CAD build for the part. Positions are in the model's coordinates, mm. Face numbers are marked on the shaded views. Coordinates: 2 decimals unless noted, no trailing zeros. Loops run counter-clockwise (first coordinate to the right, second up) from the corner with the lowest first, then second, coordinate; pieces in that order, holes last. Notation, with made-up numbers: (-33, -11) - (-29, -11) arc R22 cw to (-29, 4) - close; hole circle Ø10 at (8, 27). An arc over 180 degrees is marked (long way). Put each result on its own line as item: value.
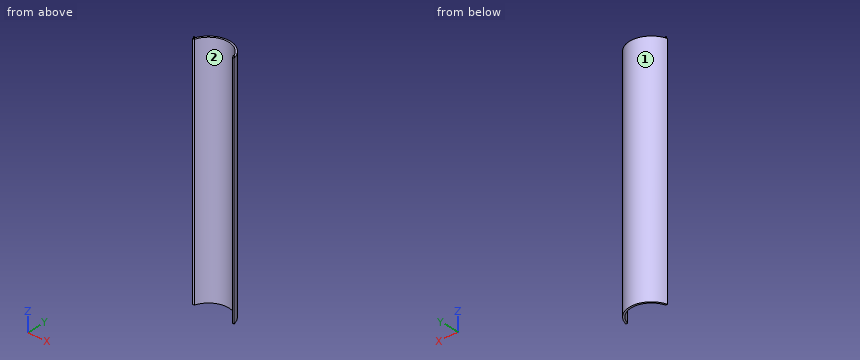
Autodesk Inventor part; units mm, degrees
ref_plane "YZ Plane" through (0, 0, 0) normal (1, 0, 0) x (0, 1, 0)
ref_plane "XZ Plane" through (0, 0, 0) normal (0, 1, 0) x (-1, 0, 0)
ref_plane "XY Plane" through (0, 0, 0) normal (0, 0, 1) x (1, 0, 0)
sketch "Sketch1" plane through (0, 0, 0) normal (0, 0, 1) x (1, 0, 0)
  circle A0 centre (0, 0) radius 25.4
  circle A1 centre (0, 0) radius 23.4
  dimension "d0" = 50.8
  dimension "d1" = 2
extrude "Extrusion1" add sketch "Sketch1" against normal blind 274
sketch "Sketch2" plane through (0, 0, 0) normal (0, 0, 1) x (1, 0, 0)
  line L0 (-25.4, 6.35) -> (25.4, 6.35)
  line L1 (25.4, 6.35) -> (25.4, -25.4)
  line L2 (25.4, -25.4) -> (-25.4, -25.4)
  line L3 (-25.4, -25.4) -> (-25.4, 6.35)
  circle A0 centre (0, 0) radius 25.4
  line L4 (0, 25.4) -> (0, -25.4)
  point P0 (-24.5934, 6.35)
  point P1 (24.5934, 6.35)
  dimension "d6" = 25.4
  dimension "d7" = 25.4
  dimension "d8" = 25.4
  dimension "d9" = 19.05
extrude "Extrusion2" cut sketch "Sketch2" against normal through all contours L0 L4 A0 | L0 A0 L4 picked at (-1.884, -14.6044) picked at (1.884, -14.6044)
sketch "Sketch3" plane through (0, 0, 0) normal (0, 0, 1) x (1, 0, 0)
  line L0 (22.5219, 6.35) -> (24.5934, 6.35)
  line L1 (23.5577, 6.35) -> (23.5577, 9.4971)
  arc A0 (24.5934, 6.35) -> (-24.5934, 6.35) centre (0, 0) ccw
  circle A1 centre (23.5577, 6.85) radius 0.5
  line L2 (0, 25.4) -> (0, 6.35) construction
  circle A2 centre (-23.5577, 6.85) radius 0.5
  dimension "d12" = 1
  dimension "d13" = 0.5
extrude "Extrusion3" add sketch "Sketch3" along normal blind 2 contours A1 L1 | L1 A1 | A2
properties part number "PCB Tray Top_3DPrint"
Q1. Slice it at A-A, the plane y = 20. Give the cut face in (x, z), then the cut area to 3 significant figures.
Determined:
outline: (-15.66, -274) - (-12.15, -274) - (-12.15, 0) - (-15.66, 0) - close; (12.15, -274) - (15.66, -274) - (15.66, 0) - (12.15, 0) - close
area: 1,920 mm2
Q2. Pin check, flat tips, straight feed: pin 1 Ø3 at (y, z) = (12.5, -99.5) entering from -X; pin 2 Ø5 at (x, z) = (-7.5, -145) entering from -Y; pin 3 Ø2 at (x, y) = (-15, 16.5) entering from +Z (3 decimals); pin 4 Ø5 at (x, z) = (-13.5, -197) entering from -Y. Stop position of each tip, or through.
Determined:
pin 1: x = -22.89
pin 2: y = 21.16
pin 3: through
pin 4: y = 17.08
Q3. Slice it at C-C, the plane x = -3. Give the cut face in (y, z).
Determined:
outline: (23.21, -274) - (25.22, -274) - (25.22, 0) - (23.21, 0) - close
Q4. Slice it at B-B, the plane z = -170. Give the cut face in (x, y), then the cut area to 3 significant figures.
Determined:
outline: (-24.59, 6.35) - (-22.52, 6.35) arc R23.4 cw to (22.52, 6.35) - (24.59, 6.35) arc R25.4 ccw to start
area: 128 mm2
Q5. Wall check: L1, parallel to Z at x = -4.5, y = 23.5; L2, parallel to X at y = 17.75, z = -30; L3, parallel to X at y = 8.5, z = -115. Give the ranges that are in metal, low to high. Write a range as from..to.
Determined:
L1: -274..0
L2: -18.17..-15.25, 15.25..18.17
L3: -23.94..-21.8, 21.8..23.94
Q6. Mould opens along X. For the marked faces 1 and 2 say: +X half, -X half, draft (parallel to the pull), parting line (faces both ways), or undercut.
Determined:
face 1: parting line
face 2: undercut
